Model file for the job. Use its own axes, mm. Round coordinates to 2 decimals unless told otherwise and drop trailing zeros. Loops run counter-clockwise (first coordinate to the right, second up) from the corner with the lowest first, then second, coordinate; pieces in that order, holes last. Notation, with made-up numbers: M 55.5,68 L 96.5,68 A26 ccw 96.5,87 Z; hole C 27,22 d4. An arc over 180 degrees is marked long. Answer in a Markdown table with one row per item.
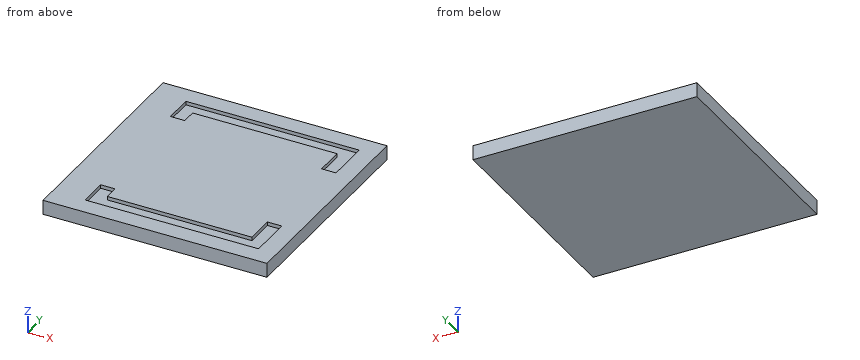
from build123d import *

# Parameters (mm, degrees)
F0_W     = 98.425
F0_H     = 98.425
F1_DEPTH = 3.175
F3_DEPTH = 1.5875


# Not quite as in the source:
# - a pattern or mirror of a feature is missing from the dataset's text; its kind, count and spacing are read off the source's solid


with BuildPart() as f1:
    # F0 (on Top) → F1 (new body, symmetric)
    with BuildSketch(Plane.XY):
        Rectangle(F0_W, F0_H)
    extrude(amount=F1_DEPTH, both=True)

    # F2 (on face) → F3 (cut, symmetric)
    with BuildSketch(Plane.XY.offset(3.175)):
        Polygon((41.275, 22.225), (41.275, 41.275), (-34.925, 41.275), (-34.925, 28.575), (-28.575, 28.575), (-28.575, 34.925), (34.925, 34.925), (34.925, 22.225), align=None)
    f3 = extrude(amount=F3_DEPTH, both=True, mode=Mode.SUBTRACT)

    # F3_copies: F3 across plane
    add(f3.mirror(Plane(origin=(0, 0, 0), x_dir=(0, 0, -1), z_dir=(0, -1, 0))), mode=Mode.SUBTRACT)


solid = f1.part
1. Saw through at A-A (x = 3.5). Write the cut outline in (y, z) (1 decimal), and give its area (3 significant figures).
Verdict:
| item | result |
|---|---|
| outline | M -49.2,-3.2 L 49.2,-3.2 L 49.2,3.2 L 41.3,3.2 L 41.3,1.6 L 34.9,1.6 L 34.9,3.2 L -34.9,3.2 L -34.9,1.6 L -41.3,1.6 L -41.3,3.2 L -49.2,3.2 Z |
| area | 605 mm² |
2. Saw through at B-B (y = 40). Write the cut outline in (x, z) (1 decimal).
Verdict:
| item | result |
|---|---|
| outline | M -49.2,-3.2 L 49.2,-3.2 L 49.2,3.2 L 41.3,3.2 L 41.3,1.6 L -34.9,1.6 L -34.9,3.2 L -49.2,3.2 Z |
3. Wall check: probe 1 along Y at (x, z) = (-28, 2.75) (1 decimal); probe 2 along X at (y, z) = (-29, 2) (1 decimal); probe 3 along X at (y, z) = (38, 2.5) (1 decimal). Give the ranges that are in metal, low to high.
Verdict:
| item | result |
|---|---|
| probe 1 | y = -49.2 to -41.3, -34.9 to 34.9, 41.3 to 49.2 |
| probe 2 | x = -49.2 to -34.9, -28.6 to 34.9, 41.3 to 49.2 |
| probe 3 | x = -49.2 to -34.9, 41.3 to 49.2 |
4. Saw through at C-C (y = -25.5). Write the cut outline in (x, z) (1 decimal), and give its area (3 significant figures).
Verdict:
| item | result |
|---|---|
| outline | M -49.2,-3.2 L 49.2,-3.2 L 49.2,3.2 L 41.3,3.2 L 41.3,1.6 L 34.9,1.6 L 34.9,3.2 L -49.2,3.2 Z |
| area | 615 mm² |
